The figure shows three views and two pictorial views of one solid part (mm, origin at its lowest corner). Answer the questions. Round coordinates to 2 decimals unless told otherwise and drop trailing zeros. Write each loop counter-clockwise with the first axis right and the second up, starting at its lowest first coordinate (ties: lowest second). Pieces come first, ordered by that corner, then holes. Notation, with made-up numbers: M 86,-26.75 L 145,-26.75 A22 ccw 145,4.25 Z; hole C 73,47 d1. An arc over 180 degrees is marked long. Answer in a Markdown table with one row per item.
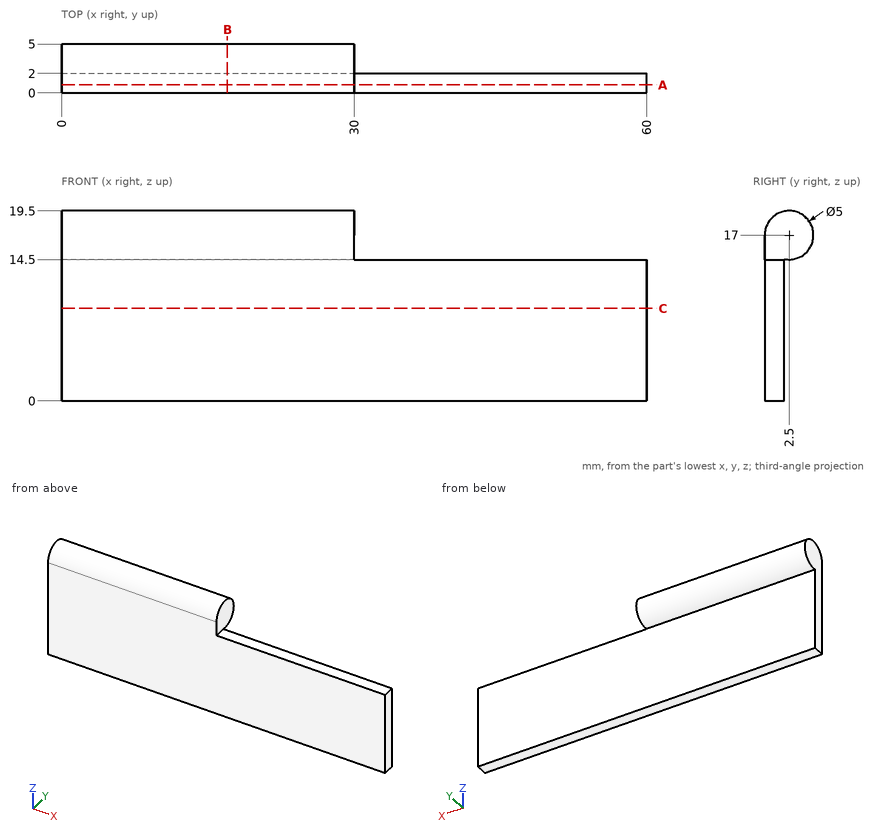
1. The part is cut by section A-A (y = 0.8). Determine the outline of the cut face in (x, z), plus the area to 4 significant figures.
Calculated:
| item | result |
|---|---|
| outline | M 0,0 L 60,0 L 60,14.5 L 30,14.5 L 30,18.83 L 0,18.83 Z |
| area | 1,000 mm² |
2. Consider line 1 along X through (y, z) = (0.25, 17); line 2 along Y through (x, z) = (24.5, 7.25); line 3 along Z through (x, y) = (46, 1.7). Determine where each line is inside the solid, lowest interval first. Write a range as from..to.
Calculated:
| item | result |
|---|---|
| line 1 | x = 0..30 |
| line 2 | y = 0..2 |
| line 3 | z = 0..14.5 |
3. The part is cut by section B-B (x = 17). Determine the outline of the cut face in (y, z), plus the area to 3 significant figures.
Calculated:
| item | result |
|---|---|
| outline | M 0,0 L 2,0 L 2,14.55 A2.5 ccw long 0,17 Z |
| area | 50.0 mm² |
4. Given pin 1 (2 mm diameter, centred on x = 21.5, z = 14, fed in from +Y); pin 2 (4 mm diameter, centred on x = 8, z = 9, fed in from +Y); pin 3 (2.5 mm diameter, centred on y = 2, z = 18, fed in from +X), each flat-ended and moving along its own axis, determine where each tip first touches the part or whether it passes through.
Calculated:
| item | result |
|---|---|
| pin 1 | stops at y = 4 |
| pin 2 | stops at y = 2 |
| pin 3 | stops at x = 30 |
5. The part is cut by section C-C (z = 9.5). Determine the outline of the cut face in (x, y).
Calculated:
| item | result |
|---|---|
| outline | M 0,0 L 60,0 L 60,2 L 0,2 Z |
